Geometry: final body of the model. Coordinates: model frame, mm. Face numbers are marked on the shaded views. Give positions to 0.01 mm unless a question says otherwise; leave off trailing zeros. Loops run counter-clockwise (first coordinate to the right, second up) from the corner with the lowest first, then second, coordinate; pieces in that order, holes last. Notation, with made-up numbers: (64.25, 88) -> (104.25, 88) arc R9 ccw to (104.25, 99) -> close; hole circle Ø7 at (14.5, 3). An arc over 180 degrees is marked (long way). Answer in a Markdown table with one row per item. Add a question column.
1) First-contact query: P1, Ø1, axis at x = 26, y = 4, coming from the +Z side; P2, Ø1.6, axis at x = 23.5, y = 3, coming from the +Z side; P3, Ø1.5, axis at x = -24.5, y = 1.5, coming from the +Z side. Flat tips, straight axial feed; report the tip coordinate or a pass-through.
2) Section query A-A (z = -50.8). Return the cut outline in (x, y).
3) Section query D-D (x = 44.5). Return the cut outline in (y, z).
4) Section query C-C (y = 1.5). Give the number of separate pieces and of enclosed holes in the cut face, plus the area to 3 significant figures.
5) Line query: line 1 (X direction, y = 5.25, z = -33); line 2 (X direction, y = 4, z = 12); line 3 (X direction, y = 2.5, z = -53.5). Output: solid intervals per line, ascending. Write a range as from..to.
6) Draft query along Y for the marked faces 1 and 2. Return one class per face: +Y half, -Y half, draft (parallel to the pull), parting line (faces both ways), or undercut.
7) Section query B-B (x = -38.1). Return the cut outline in (y, z), plus the area to 3 significant figures.
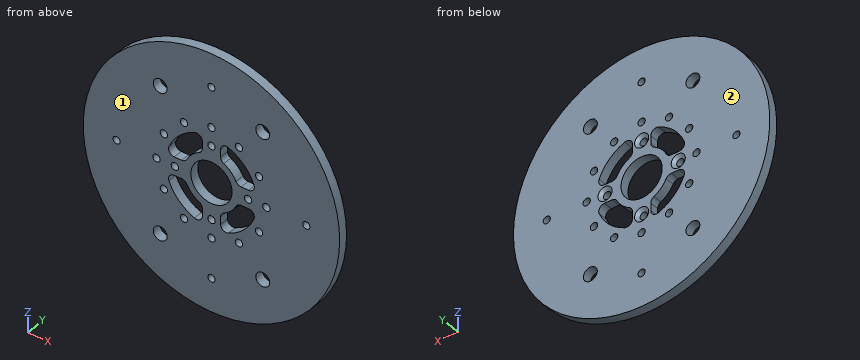
```python
from build123d import *

# Parameters (mm, degrees)
SKETCH1_R                                          = 88.9
BOSS_EXTRUDE1_DEPTH                                = 6.35
SKETCH2_R                                          = 14.2875
CUT_EXTRUDE1_DEPTH                                 = 7.35
CSK_FOR_10_FLAT_HEAD_MACHINE_SCREW_100_D           = 5.1054
CSK_FOR_10_FLAT_HEAD_MACHINE_SCREW_100_CSINK_D     = 9.779
CSK_FOR_10_FLAT_HEAD_MACHINE_SCREW_100_CSINK_ANGLE = 100
F_9_0_196_DIAMETER_HOLE1_D                         = 4.9784
F_1_4_20_TAPPED_HOLE1_D                            = 5.1054
CUT_EXTRUDE3_DEPTH                                 = 6.35
SKETCH17_R                                         = 4.826
CUT_EXTRUDE4_DEPTH                                 = 7.35


with BuildPart() as part:
    # Sketch1 → Boss-Extrude1 (new body)
    with BuildSketch(Plane(origin=(0, 0, 0), x_dir=(1, 0, 0), z_dir=(0, 1, 0))):
        Circle(SKETCH1_R)
    extrude(amount=BOSS_EXTRUDE1_DEPTH)

    # Sketch2 → Cut-Extrude1 (cut, through all)
    with BuildSketch(Plane(origin=(0, 6.35, 0), x_dir=(1, 0, 0), z_dir=(0, 1, 0))):
        Circle(SKETCH2_R)
    extrude(amount=-CUT_EXTRUDE1_DEPTH, mode=Mode.SUBTRACT)

    # CSK for #10 Flat Head Machine Screw (100)1 (through all)
    with Locations(Plane(origin=(0, 6.35, 0), x_dir=(1, 0, 0), z_dir=(0, 1, 0))):
        with Locations((0, 25.4), (25.4, 0), (0, -25.4), (-25.4, 0)):
            CounterSinkHole(CSK_FOR_10_FLAT_HEAD_MACHINE_SCREW_100_D / 2, CSK_FOR_10_FLAT_HEAD_MACHINE_SCREW_100_CSINK_D / 2, counter_sink_angle=CSK_FOR_10_FLAT_HEAD_MACHINE_SCREW_100_CSINK_ANGLE)

    # #9 (0.196) Diameter Hole1 (through all)
    with Locations(Plane(origin=(0, 6.35, 0), x_dir=(1, 0, 0), z_dir=(0, 1, 0))):
        with Locations((0, 65.786), (65.786, 0), (0, -65.786), (-65.786, 0)):
            Hole(F_9_0_196_DIAMETER_HOLE1_D / 2)

    # 1/4-20 Tapped Hole1 (through all)
    with Locations(Plane(origin=(0, 6.35, 0), x_dir=(1, 0, 0), z_dir=(0, 1, 0))):
        with Locations((0, 38.1), (19.05, 32.995567884), (32.995567884, 19.05), (38.1, 0), (32.995567884, -19.05), (19.05, -32.995567884), (0, -38.1), (-19.05, -32.995567884), (-32.995567884, -19.05), (-38.1, 0), (-32.995567884, 19.05), (-19.05, 32.995567884)):
            Hole(F_1_4_20_TAPPED_HOLE1_D / 2)

    # Sketch16 → Cut-Extrude3 (cut)
    with BuildSketch(Plane(origin=(0, 6.35, 0), x_dir=(1, 0, 0), z_dir=(0, 1, 0))):
        with BuildLine():
            Line((20.576351717, 6.35), (25.793821935, 6.35))
            ThreePointArc((25.793821935, 6.35), (29.080259161, 8.09382148), (29.47865364, 11.792857143))
            ThreePointArc((29.47865364, 11.792857143), (22.450640303, 22.450640303), (11.792857143, 29.47865364))
            ThreePointArc((11.792857143, 29.47865364), (8.09382148, 29.080259161), (6.35, 25.793821935))
            Line((6.35, 25.793821935), (6.35, 20.576351717))
            ThreePointArc((6.35, 20.576351717), (6.941490818, 18.491862096), (8.539655172, 17.02870487))
            ThreePointArc((8.539655172, 17.02870487), (13.470384182, 13.470384182), (17.02870487, 8.539655172))
            ThreePointArc((17.02870487, 8.539655172), (18.491862096, 6.941490818), (20.576351717, 6.35))
        make_face()
        with BuildLine():
            Line((6.35, -20.576351717), (6.35, -25.793821935))
            ThreePointArc((6.35, -25.793821935), (8.09382148, -29.080259161), (11.792857143, -29.47865364))
            ThreePointArc((11.792857143, -29.47865364), (22.450640303, -22.450640303), (29.47865364, -11.792857143))
            ThreePointArc((29.47865364, -11.792857143), (29.080259161, -8.09382148), (25.793821935, -6.35))
            Line((25.793821935, -6.35), (20.576351717, -6.35))
            ThreePointArc((20.576351717, -6.35), (18.491862096, -6.941490818), (17.02870487, -8.539655172))
            ThreePointArc((17.02870487, -8.539655172), (13.470384182, -13.470384182), (8.539655172, -17.02870487))
            ThreePointArc((8.539655172, -17.02870487), (6.941490818, -18.491862096), (6.35, -20.576351717))
        make_face()
        with BuildLine():
            Line((-20.576351717, -6.35), (-25.793821935, -6.35))
            ThreePointArc((-25.793821935, -6.35), (-29.080259161, -8.09382148), (-29.47865364, -11.792857143))
            ThreePointArc((-29.47865364, -11.792857143), (-22.450640303, -22.450640303), (-11.792857143, -29.47865364))
            ThreePointArc((-11.792857143, -29.47865364), (-8.09382148, -29.080259161), (-6.35, -25.793821935))
            Line((-6.35, -25.793821935), (-6.35, -20.576351717))
            ThreePointArc((-6.35, -20.576351717), (-6.941490818, -18.491862096), (-8.539655172, -17.02870487))
            ThreePointArc((-8.539655172, -17.02870487), (-13.470384182, -13.470384182), (-17.02870487, -8.539655172))
            ThreePointArc((-17.02870487, -8.539655172), (-18.491862096, -6.941490818), (-20.576351717, -6.35))
        make_face()
        with BuildLine():
            Line((-6.35, 20.576351717), (-6.35, 25.793821935))
            ThreePointArc((-6.35, 25.793821935), (-8.09382148, 29.080259161), (-11.792857143, 29.47865364))
            ThreePointArc((-11.792857143, 29.47865364), (-22.450640303, 22.450640303), (-29.47865364, 11.792857143))
            ThreePointArc((-29.47865364, 11.792857143), (-29.080259161, 8.09382148), (-25.793821935, 6.35))
            Line((-25.793821935, 6.35), (-20.576351717, 6.35))
            ThreePointArc((-20.576351717, 6.35), (-18.491862096, 6.941490818), (-17.02870487, 8.539655172))
            ThreePointArc((-17.02870487, 8.539655172), (-13.470384182, 13.470384182), (-8.539655172, 17.02870487))
            ThreePointArc((-8.539655172, 17.02870487), (-6.941490818, 18.491862096), (-6.35, 20.576351717))
        make_face()
    extrude(amount=-CUT_EXTRUDE3_DEPTH, mode=Mode.SUBTRACT)

    # Sketch17 → Cut-Extrude4 (cut, through all)
    with BuildSketch(Plane(origin=(0, 6.35, 0), x_dir=(1, 0, 0), z_dir=(0, 1, 0))):
        with Locations((-35.56, -50.8)):
            Circle(SKETCH17_R)
        with Locations((-35.56, 50.8)):
            Circle(SKETCH17_R)
        with Locations((35.56, -50.8)):
            Circle(SKETCH17_R)
        with Locations((35.56, 50.8)):
            Circle(SKETCH17_R)
    extrude(amount=-CUT_EXTRUDE4_DEPTH, mode=Mode.SUBTRACT)


solid = part.part
```
Evaluation:
| question | item | result |
|---|---|---|
| 1 | P1 | z = 85.16 |
| 1 | P2 | z = 85.95 |
| 1 | P3 | z = 85.67 |
| 2 | outline | (-72.96, 0) -> (-40.39, 0) -> (-40.39, 6.35) -> (-72.96, 6.35) -> close; (-30.73, 0) -> (30.73, 0) -> (30.73, 6.35) -> (-30.73, 6.35) -> close; (40.39, 0) -> (72.96, 0) -> (72.96, 6.35) -> (40.39, 6.35) -> close |
| 3 | outline | (0, -76.96) -> (6.35, -76.96) -> (6.35, 76.96) -> (0, 76.96) -> close |
| 4 | separate pieces | 1 |
| 4 | enclosed holes | 29 |
| 4 | area | 22,200 mm² |
| 5 | line 1 | -82.55..-21.6, -16.5..16.5, 21.6..82.55 |
| 5 | line 2 | -88.09..-29.39, -14.8..-7.75, 7.75..14.8, 29.39..88.09 |
| 5 | line 3 | -71..-39.56, -31.56..31.56, 39.56..71 |
| 6 | face 1 | -Y half |
| 6 | face 2 | +Y half |
| 7 | outline | (0, -80.32) -> (6.35, -80.32) -> (6.35, -54.9) -> (0, -54.9) -> close; (0, -46.7) -> (6.35, -46.7) -> (6.35, -2.55) -> (0, -2.55) -> close; (0, 2.55) -> (6.35, 2.55) -> (6.35, 46.7) -> (0, 46.7) -> close; (0, 54.9) -> (6.35, 54.9) -> (6.35, 80.32) -> (0, 80.32) -> close |
| 7 | area | 883 mm² |
